The model under review builds one solid part; all positions refer to its coordinate system, in mm. A direction names the side the tool comes from. Coordinates: 2 decimals unless noted, no trailing zeros. Loops run counter-clockwise (first coordinate to the right, second up) from the corner with the lowest first, then second, coordinate; pieces in that order, holes last. Notation, with made-up numbers: (73.5, -31) - (130.5, -31) arc R15 cw to (130.5, -20) - close; hole circle Ø9 at (46, -4). An arc over 180 degrees is marked (long way). Answer in a Markdown table with one row per item. Add a question column.
(1) Mouldability with a two-part tool opening along Z and no side actions: class faces 3 (the flat face through (0, 0, 0)), 4 (the cylindrical face through (30.5, 6.5, 12.6)), 5 (the cylindrical face through (-33.75, 8.29, 0.13)), 6 (the cylindrical face through (32.907, 4.93, -10.363)) as +Z half, -Z half, draft (parallel to the pull), parting line (faces both ways), or undercut.
(2) We need section A-A on z = 0. Write out the cut boundary in (x, y).
(3) For P1, Ø2, axis at x = 9.5, z = -18, coming from the +Y side; P2, Ø4, axis at y = 8.5, z = -5.5, coming from the -X side; P3, Ø1.5, axis at y = 7.5, z = -20.5, coming from the -X side, all flat-tipped, find the tip position at first contact; note any pin that passes through.
(4) We need section D-D on z = 27.5. Write out the cut boundary in (x, y).
(5) For line 1 along Z through (x, y) = (0, 7.5); line 2 along Y through (x, z) = (34, 0), list the stretches that pass through material, from the lowest coordinate up.
(6) Machinability: for faces 1 (the cylindrical face through (33.73, 8.29, 0.13)), 2 (the flat face through (0, 3, 0)), which of the approach directions +Z, -Z, +X, -X, +Y, -Y give a long, thin tool a straight path to every point of the face, cutting with its end or side? Answer none if there is none.
(7) We need section C-C on x = 0. Write out the cut boundary in (y, z).
from build123d import *

# Parameters (mm, degrees)
SKETCH1_R               = 34.5
BOSS_EXTRUDE1_DEPTH     = 10
SKETCH2_R               = 33
CUT_EXTRUDE1_DEPTH      = 7
SKETCH3_R               = 1
CUT_EXTRUDE2_DEPTH      = 71.585008529
CUT_EXTRUDE2_DEPTH_BACK = 1


with BuildPart() as part:
    # Sketch1 → Boss-Extrude1 (new body)
    with BuildSketch(Plane(origin=(0, 0, 0), x_dir=(1, 0, 0), z_dir=(0, 1, 0))):
        Circle(SKETCH1_R)
    extrude(amount=BOSS_EXTRUDE1_DEPTH)

    # Sketch2 → Cut-Extrude1 (cut)
    with BuildSketch(Plane(origin=(0, 10, 0), x_dir=(1, 0, 0), z_dir=(0, 1, 0))):
        Circle(SKETCH2_R)
    extrude(amount=-CUT_EXTRUDE1_DEPTH, mode=Mode.SUBTRACT)

    # Sketch3 → Cut-Extrude2 (cut, two sides)
    with BuildSketch(Plane(origin=(-36.085008529, 0, 0), x_dir=(0, 0, -1), z_dir=(1, 0, 0))) as cut_extrude2_sk:
        with Locations((0, 7.3)):
            Circle(SKETCH3_R)
    extrude(amount=CUT_EXTRUDE2_DEPTH, mode=Mode.SUBTRACT)
    extrude(cut_extrude2_sk.sketch, amount=-CUT_EXTRUDE2_DEPTH_BACK, mode=Mode.SUBTRACT)


solid = part.part
Outcome:
| question | item | result |
|---|---|---|
| 1 | face 3 | draft |
| 1 | face 4 | undercut |
| 1 | face 5 | undercut |
| 1 | face 6 | parting line |
| 2 | outline | (-34.5, 0) - (34.5, 0) - (34.5, 6.3) - (33, 6.3) - (33, 3) - (-33, 3) - (-33, 6.3) - (-34.5, 6.3) - close; (-34.5, 8.3) - (-33, 8.3) - (-33, 10) - (-34.5, 10) - close; (33, 8.3) - (34.5, 8.3) - (34.5, 10) - (33, 10) - close |
| 3 | P1 | y = 3 |
| 3 | P2 | x = -34.32 |
| 3 | P3 | x = -28.29 |
| 4 | outline | (-20.83, 0) - (20.83, 0) - (20.83, 10) - (18.24, 10) - (18.24, 3) - (-18.24, 3) - (-18.24, 10) - (-20.83, 10) - close |
| 5 | line 1 | -34.5 to -33, 33 to 34.5 |
| 5 | line 2 | 0 to 6.3, 8.3 to 10 |
| 6 | face 1 | +X, -X |
| 6 | face 2 | +Y |
| 7 | outline | (0, -34.5) - (10, -34.5) - (10, -33) - (3, -33) - (3, 33) - (10, 33) - (10, 34.5) - (0, 34.5) - close |
